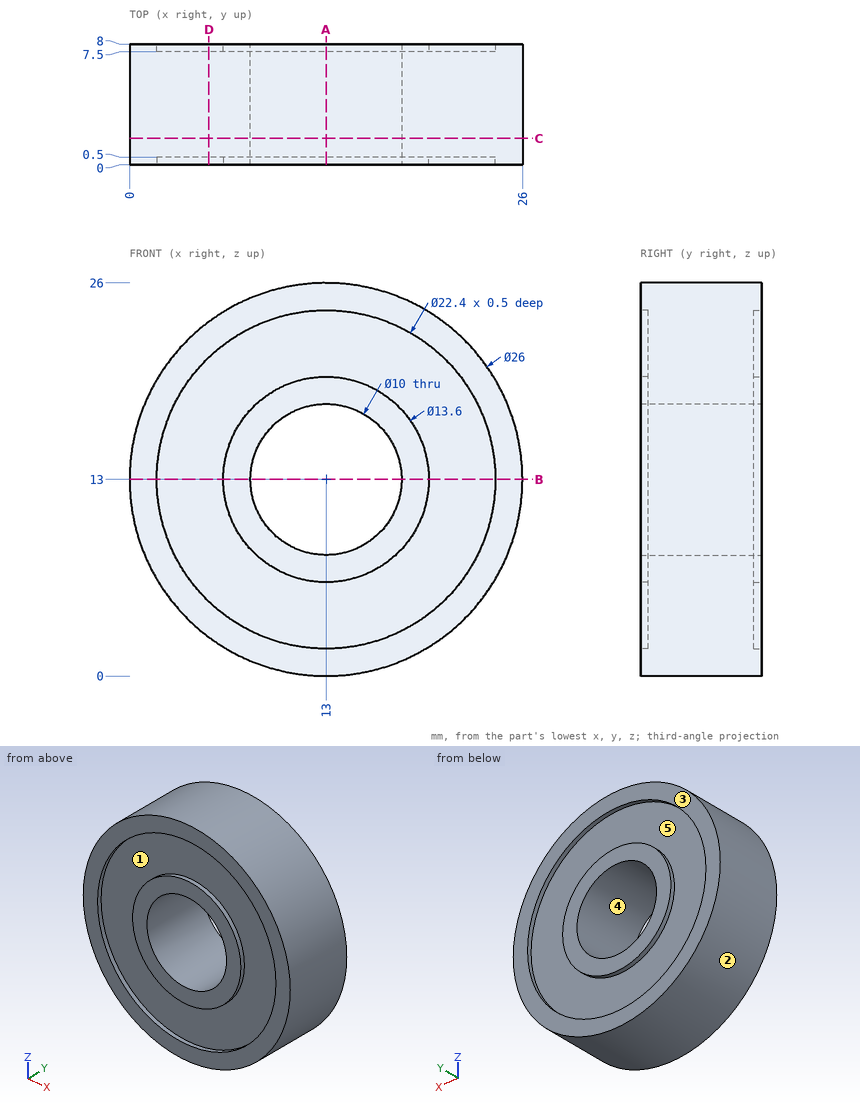
Job drawing, mm, ordinate dimensions from the low corner. One solid piece. A direction names the side the tool comes from. Coordinates: 2 decimals unless noted, no trailing zeros. Loops run counter-clockwise (first coordinate to the right, second up) from the corner with the lowest first, then second, coordinate; pieces in that order, holes last. Notation, with made-up numbers: (64, 55.25) - (102, 55.25) arc R26 cw to (102, 76.25) - close; hole circle Ø4 at (82.25, 42). An arc over 180 degrees is marked (long way). Answer as a JSON object with one key per item and string values. Group by question number.
(1) Cut at A-A (x = 13). Give the cut face in (y, z).
(2) Cut at D-D (x = 5.25). Give the cut face in (y, z), then the cut area to 3 significant figures.
(3) Tool access for the marked faces 4 and 5: list every direction of +Z, -Z, +X, -X, +Y, -Y with a clear straight run to the whole face (end or side of a thin tool).
(4) Cut at C-C (y = 1.75). Give the cut face in (x, z).
(5) Probe line 1 along Z through (x, y) = (13, 7.9); line 2 along Z through (x, y) = (13, 2); line 3 along Y through (x, z) = (11, 4.5). List the from-to ranges inside material, lowest first.
(6) Flat gauge pins, fed straight in: pin 1 (2 mm diameter, centred on y = 4.5, z = 17.5, fed in from -X); pin 2 (4 mm diameter, centred on y = 6.5, z = 22.5, fed in from -X); pin 3 (3 mm diameter, centred on x = 10.5, y = 3, fed in from +Z). Where does each tip first touch, or does it go through?
(7) Two-plate mould, pull along Z, no slides. Class the marked faces 1, 2 and 3: released by +Z, released by -Z, zero draft, split by the parting line, or undercut.
(8) Cut at B-B (z = 13). Give the cut face in (x, y), then the cut area to 3 significant figures.
Geometry says:
{
 "1": {"outline": "(0, 0) - (8, 0) - (8, 1.8) - (7.5, 1.8) - (7.5, 6.2) - (8, 6.2) - (8, 8) - (0, 8) - (0, 6.2) - (0.5, 6.2) - (0.5, 1.8) - (0, 1.8) - close; (0, 18) - (8, 18) - (8, 19.8) - (7.5, 19.8) - (7.5, 24.2) - (8, 24.2) - (8, 26) - (0, 26) - (0, 24.2) - (0.5, 24.2) - (0.5, 19.8) - (0, 19.8) - close"},
 "2": {"outline": "(0, 2.56) - (8, 2.56) - (8, 4.91) - (7.5, 4.91) - (7.5, 21.09) - (8, 21.09) - (8, 23.44) - (0, 23.44) - (0, 21.09) - (0.5, 21.09) - (0.5, 4.91) - (0, 4.91) - close", "area": "151 mm^2"},
 "3": {"face 4": "+Y, -Y", "face 5": "+Y"},
 "4": {"outline": "circle Ø26 at (13, 13); hole circle Ø10 at (13, 13)"},
 "5": {"line 1": "z = 0 to 1.8, 6.2 to 8, 18 to 19.8, 24.2 to 26", "line 2": "z = 0 to 8, 18 to 26", "line 3": "y = 0.5 to 7.5"},
 "6": {"pin 1": "stops at x = 0.48", "pin 2": "stops at x = 2.38", "pin 3": "stops at z = 25.96"},
 "7": {"face 1": "undercut", "face 2": "split by the parting line", "face 3": "zero draft"},
 "8": {"outline": "(0, 0) - (1.8, 0) - (1.8, 0.5) - (6.2, 0.5) - (6.2, 0) - (8, 0) - (8, 8) - (6.2, 8) - (6.2, 7.5) - (1.8, 7.5) - (1.8, 8) - (0, 8) - close; (18, 0) - (19.8, 0) - (19.8, 0.5) - (24.2, 0.5) - (24.2, 0) - (26, 0) - (26, 8) - (24.2, 8) - (24.2, 7.5) - (19.8, 7.5) - (19.8, 8) - (18, 8) - close", "area": "119 mm^2"}
}
